Here's how the part is built. I have some questions about the finished solid (model axes, mm). A direction names the side the tool comes from. Coordinates: 2 decimals unless noted, no trailing zeros. Write each loop counter-clockwise with the first axis right and the second up, starting at its lowest first coordinate (ties: lowest second). Pieces come first, ordered by that corner, then holes. Notation, with made-up numbers: (18.5, 31.5) -> (72.5, 31.5) arc R13 ccw to (72.5, 50.5) -> close; hole circle Ø2 at (44, 21). An arc over 180 degrees is marked (long way). Use a Markdown table: item, result. Add a question column.
Item 1: If we mould it in two halves opening along Z, with no side actions, what happens to faces 4 (the flat face through (102.465, 177.475, 59.16)), 5 (the flat face through (0, 203, 0)), 6 (the cylindrical face through (5.618, 225.384, 79.575))? For each: pulls with the +Z half, pulls with the -Z half, needs draft (parallel to the pull), parting line crosses it, or undercut.
Item 2: Imagine slicing it at A-A, the plane z = 30.5. Write out the boundary of the cut face in (x, y), and give its area (3 significant figures).
Item 3: Imagine slicing it at C-C, the plane y = 227. Write out the boundary of the cut face in (x, z).
Item 4: Imagine slicing it at D-D, the plane x = 33. Write out the boundary of the cut face in (y, z), and give its area (3 significant figures).
Item 5: Will these pins go through, and if not, where does the flat tip stop? pin 1 Ø4 at (x, y) = (-55.5, 189.5) entering from -Z; pin 2 Ø8 at (y, z) = (224.5, 64.5) entering from +X; pin 3 Ø1 at (x, z) = (-48, 103) entering from -Y; pin 4 Ø5 at (y, z) = (223.5, 41.5) entering from -X.
Item 6: If I drill on line 1 along Z through (x, y) = (-79, 187.5); line 2 along X through (y, z) = (180, 78.5); line 3 along Z through (x, y) = (-21, 220), over which ranges is the centre line in solid material (lowest first)? Write a range as from..to.
Item 7: On a 3-axis mill with a long thin cutter (end or side, diameter ignored), from which of +Z, -Z, +X, -X, +Y, -Y can I reach the whole of each face in a straight line? I mean faces 1 (the cylindrical face through (70.483, 217.7, 60.184)), 2 (the cylindrical face through (1.459, 200.995, 87.048)), 3 (the cylindrical face through (-69.51, 217.88, 59.58)). Say none if no direction works.
Item 8: Imagine slicing it at B-B, the plane x = -37. Write out the boundary of the cut face in (y, z), and give its area (3 significant figures).
```python
from build123d import *

# Parameters (mm, degrees)
BOSS_EXTRUDE1_DEPTH = 120
CUT_EXTRUDE1_DEPTH  = 118
BOSS_EXTRUDE2_DEPTH = 248
CUT_EXTRUDE2_DEPTH  = 269


with BuildPart() as part:
    # Sketch1 → Boss-Extrude1 (new body)
    with BuildSketch(Plane.XY):
        with BuildLine():
            Line((-105, 181.865334795), (-100, 173.205080757))
            ThreePointArc((-100, 173.205080757), (0, 200), (100, 173.205080757))
            Line((100, 173.205080757), (105, 181.865334795))
            ThreePointArc((105, 181.865334795), (0, 210), (-105, 181.865334795))
        make_face()
    extrude(amount=BOSS_EXTRUDE1_DEPTH)

    # Sketch2 → Cut-Extrude1 (cut)
    with BuildSketch(Plane.XY.offset(119)):
        with BuildLine():
            ThreePointArc((99.632730807, 174.568951855), (0, 201), (-99.632730807, 174.568951855))
            Line((-99.632730807, 174.568951855), (-103.632778417, 181.497237548))
            Line((-103.632778417, 181.497237548), (-105, 184.581371686))
            Line((-105, 184.581371686), (38.612235753, 274.588582832))
            Line((38.612235753, 274.588582832), (105, 184.581371686))
            Line((105, 184.581371686), (103.632778417, 181.497237548))
            Line((103.632778417, 181.497237548), (99.632730807, 174.568951855))
        make_face()
    extrude(amount=-CUT_EXTRUDE1_DEPTH, mode=Mode.SUBTRACT)

    # Sketch3 → Boss-Extrude2 (add)
    with BuildSketch(Plane(origin=(0, 0, 0), x_dir=(1, 0, 0), z_dir=(0, 1, 0))):
        with BuildLine():
            ThreePointArc((-51.003018744, -40.055400821), (-69.515415438, -60), (-51.003018744, -79.944599179))
            ThreePointArc((-51.003018744, -79.944599179), (6.419962074, -79.503661207), (62.997953546, -69.67899666))
            ThreePointArc((62.997953546, -69.67899666), (70.484584562, -60), (62.997953546, -50.32100334))
            ThreePointArc((62.997953546, -50.32100334), (6.419962074, -40.496338793), (-51.003018744, -40.055400821))
        make_face()
    extrude(amount=BOSS_EXTRUDE2_DEPTH)

    # Sketch4 → Cut-Extrude2 (cut)
    with BuildSketch(Plane.XY):
        with BuildLine():
            Line((70.484584562, 187.168168606), (163.146781593, -79.750206807))
            Line((163.146781593, -79.750206807), (-229.131099013, -106.991726293))
            Line((-229.131099013, -106.991726293), (-69.515415438, 187.530282932))
            ThreePointArc((-69.515415438, 187.530282932), (0.51730445, 199.999330989), (70.484584562, 187.168168606))
        make_face()
    extrude(amount=CUT_EXTRUDE2_DEPTH, mode=Mode.SUBTRACT)


solid = part.part
```
Ans:
| question | item | result |
|---|---|---|
| 1 | face 4 | needs draft |
| 1 | face 5 | pulls with the -Z half |
| 1 | face 6 | undercut |
| 2 | outline | (-105, 181.87) -> (-100, 173.21) arc R200 cw to (100, 173.21) -> (105, 181.87) arc R210 ccw to (104.04, 182.42) -> (103.63, 181.5) -> (99.63, 174.57) arc R201 ccw to (-99.63, 174.57) -> (-103.63, 181.5) -> (-104.04, 182.42) arc R210 ccw to start |
| 2 | area | 228 mm^2 |
| 3 | outline | (-51, 40.06) arc R350 ccw to (63, 50.32) arc R10 ccw to (63, 69.68) arc R350 ccw to (-51, 79.94) arc R20 ccw to start |
| 4 | outline | (197.26, 0) -> (207.39, 0) -> (207.39, 1) -> (198.27, 1) -> (198.27, 43.92) -> (248, 43.92) -> (248, 76.08) -> (198.27, 76.08) -> (198.27, 119) -> (207.39, 119) -> (207.39, 120) -> (197.26, 120) -> close |
| 4 | area | 1,740 mm^2 |
| 5 | pin 1 | passes through |
| 5 | pin 2 | stops at x = 70.47 |
| 5 | pin 3 | stops at y = 194.03 |
| 5 | pin 4 | stops at x = -61.52 |
| 6 | line 1 | z = 0..1, 119..120 |
| 6 | line 2 | x = -103.92..-102.77, -89.45..-87.18, 87.18..89.45, 102.77..103.92 |
| 6 | line 3 | z = 39.11..80.89 |
| 7 | face 1 | +X, +Y |
| 7 | face 2 | +Y |
| 7 | face 3 | -X, +Y |
| 8 | outline | (196.55, 0) -> (206.71, 0) -> (206.71, 1) -> (197.57, 1) -> (197.57, 39.29) -> (248, 39.29) -> (248, 80.71) -> (197.57, 80.71) -> (197.57, 119) -> (206.71, 119) -> (206.71, 120) -> (196.55, 120) -> close |
| 8 | area | 2,230 mm^2 |
